Could you check a few things on this model? Use its own coordinates, in mm. A direction names the side the tool comes from. Coordinates: 2 decimals unless noted, no trailing zeros. Loops run counter-clockwise (first coordinate to the right, second up) from the corner with the lowest first, then second, coordinate; pieces in that order, holes last. Notation, with made-up numbers: (22, 45) -> (75, 45) arc R26 cw to (75, 72) -> close; hole circle Ø6 at (45, 61.5). An arc over 180 degrees is marked (long way). One line per question, with ' | ' between items.
```python
from build123d import *

# Parameters (mm, degrees)
SALIENTE_EXTRUIR1_DEPTH = 3
CROQUIS2_R              = 5.5
SALIENTE_EXTRUIR2_DEPTH = 10.4
REDONDEO3_R             = 0.2
CROQUIS4_R              = 2.5
CORTAR_EXTRUIR1_DEPTH   = 10


with BuildPart() as part:
    # Croquis1 → Saliente-Extruir1 (new body)
    with BuildSketch(Plane(origin=(0, 0, 0), x_dir=(1, 0, 0), z_dir=(0, 1, 0))):
        Polygon((0, -6.9), (5.975575286, -3.45), (5.975575286, 3.45), (0, 6.9), (-5.975575286, 3.45), (-5.975575286, -3.45), align=None)
    extrude(amount=SALIENTE_EXTRUIR1_DEPTH)

    # Croquis2 → Saliente-Extruir2 (add)
    with BuildSketch(Plane(origin=(0, 3, 0), x_dir=(1, 0, 0), z_dir=(0, 1, 0))):
        Circle(CROQUIS2_R)
    extrude(amount=SALIENTE_EXTRUIR2_DEPTH)

    # Croquis3 → Cortar-Revoluci_n17 (revolve, cut)
    with BuildSketch(Plane(origin=(0, 0, 0), x_dir=(0.866025404, 0, 0.5), z_dir=(-0.5, 0, 0.866025404))):
        with BuildLine():
            Line((-0.05505313, 13.4), (-9.065705725, 13.4))
            Line((-9.065705725, 13.4), (-9.065705725, 3))
            Line((-9.065705725, 3), (-5.242775997, 3))
            add(Edge.make_bspline(
                [(-0.05505313, 13.4), (-3.55300642, 12.195542183), (-5.129402013, 7.591757737), (-5.242775997, 3)],
                knots=[0.003430867, 0.003430867, 0.003430867, 0.003430867, 0.878426724, 0.878426724, 0.878426724, 0.878426724], degree=3))
        make_face()
    revolve(axis=Axis((0, 16.4, 0), (0, -1, 0)), mode=Mode.SUBTRACT)

    # Redondeo3
    redondeo3_edges = [part.edges().sort_by_distance(p)[0] for p in [
        (0.04767741, 13.4, 0.027526565),
    ]]
    fillet(redondeo3_edges, radius=REDONDEO3_R)

    # Croquis4 → Cortar-Extruir1 (cut)
    with BuildSketch(Plane.XZ):
        Circle(CROQUIS4_R)
    extrude(amount=-CORTAR_EXTRUIR1_DEPTH, mode=Mode.SUBTRACT)


solid = part.part
```
Q1. Imagine slicing it at B-B on z = 6. Write out the boundary of the cut face in (x, y).
Values follow:
outline: (-1.56, 0) -> (1.56, 0) -> (1.56, 3) -> (-1.56, 3) -> close
Q2. For faces 4 (the face through (-1.8, 3, 5.1)), 5 (the face through (-0.54, 4.93, -2.44)), 6 (the face through (-3.03, 1.48, 5.15)), which set-ups out of +Z, -Z, +X, -X, +Y, -Y let a thin tool reach every point of the face, with its end or its side?
Values follow:
face 4: +Y | face 5: -Y | face 6: +Z, -X, +Y, -Y
Q3. Imagine slicing it at A-A on y = 2.25. Write out the boundary of the cut face in (x, z).
Values follow:
outline: (-5.98, -3.45) -> (0, -6.9) -> (5.98, -3.45) -> (5.98, 3.45) -> (0, 6.9) -> (-5.98, 3.45) -> close; hole circle Ø5 at (0, 0)
Q4. Please list where these lines run through material, in increasing order: L1, parallel to Y at x = 4.5, z = 4; L2, parallel to X at y = 9.75, z = -1.5; L3, parallel to Z at x = 1.5, y = 8.25. Write a range as [from, to].
Values follow:
L1: y = [0, 3] | L2: x = [-3.48, -2], [2, 3.48] | L3: z = [-4.13, -2], [2, 4.13]
Q5. We'd pull the mould along Z, two halves only. Please class faces 1 (the face through (0, 10, 0)), 2 (the face through (3.03, 1.48, -5.15)), 3 (the face through (-5.976, 1, 0)): released by +Z, released by -Z, zero draft, split by the parting line, or undercut.
Values follow:
face 1: undercut | face 2: released by -Z | face 3: zero draft
Q6. For pin 1 (4 mm diameter, centred on x = 0.5, y = 8, fed in from -Z); pin 2 (3 mm diameter, centred on x = -3, y = 9.5, fed in from +Z); pin 3 (2.5 mm diameter, centred on x = -0.5, z = -0.5, fed in from -Y), each with a flat end and sliding along its axis, tell me the tip position at first contact or that it passes through.
Values follow:
pin 1: stops at z = -4.94 | pin 2: stops at z = 3.87 | pin 3: stops at y = 10
